The model under review builds one solid part; all positions refer to its coordinate system, in mm. A direction names the side the tool comes from. Round coordinates to 2 decimals unless told otherwise and drop trailing zeros. Order: outer loops, then holes, each group sorted by start corner. A loop starts at its lowest first (then second) coordinate and runs counter-clockwise, first axis right, second up. Notation, with made-up numbers: M -36.5,-34 L -2.5,-34 A27 cw -2.5,-18 Z; hole C -35,36.25 d6. An arc over 180 degrees is marked long. Answer as a JSON object with one key per item and string values. Group by question number.
1) The part is to be moulded in two halves that separate along X. For faces 3 (the cylindrical face through (12.932, -5.362, 76.415)), 4 (the cylindrical face through (-6.1, -0.2, 22.64)), 5 (the flat face through (0, 0, 0)), say which applies: +X half, -X half, draft (parallel to the pull), parting line (faces both ways), or undercut.
2) For faces 1 (the cylindrical face through (-2.17, -9.76, 167.32)), 2 (the flat face through (0, 0, 210)), list the 3-axis set-ups (+Z, -Z, +X, -X, +Y, -Y) from which the entire face can be reached by the end or side of a thin tool; tool diameter is ignored.
3) Consider section C-C, the plane z = 147. Write out the cut boundary in (x, y), then the cut area to 3 significant figures.
4) Consider section A-A, the plane x = 0. Write out the cut boundary in (y, z), then the cut area to 3 significant figures.
5) To check wall thickness, follow line 1 (Z direction, x = -1.5, y = -1.5); line 2 (Z direction, x = -1.75, y = -12.5); line 3 (X direction, y = 11.25, z = 19.5). State the ranges of each line that lie inside material, in increasing order.
6) Consider section B-B, the plane y = 5. Write out the cut boundary in (x, z) (3 decimals), then the cut area to 3 significant figures.
7) Consider section D-D, the plane y = -4.5. Write out the cut boundary in (x, z), then the cut area to 3 significant figures.
8) Insertion check: pin 1 Ø6 at (x, z) = (-6, 39.5) entering from +Y; pin 2 Ø6 at (x, z) = (8.5, 99) entering from +Y; pin 3 Ø1.5 at (x, z) = (6.5, 184) entering from -Y; pin 4 Ø10.5 at (x, z) = (0.39, 22.24) entering from -Y. Each pin has a flat end and moves straight along its axis. Give the tip position at first contact, or say it passes through.
```python
from build123d import *

# Parameters (mm, degrees)
SKETCH_R     = 14
PAD_DEPTH    = 155
SKETCH001_R  = 10
PAD001_DEPTH = 25
SKETCH002_R  = 8
PAD002_DEPTH = 30
SKETCH003_R  = 6.5
POCKET_DEPTH = 14


with BuildPart() as part:
    # Sketch → Pad (new body)
    with BuildSketch(Plane.XY):
        Circle(SKETCH_R)
    extrude(amount=PAD_DEPTH)

    # Sketch001 (on Face3 of Pad) → Pad001 (join)
    with BuildSketch(Plane.XY.offset(155)):
        Circle(SKETCH001_R)
    extrude(amount=PAD001_DEPTH)

    # Sketch002 (on Face5 of Pad001) → Pad002 (join)
    with BuildSketch(Plane.XY.offset(180)):
        Circle(SKETCH002_R)
    extrude(amount=PAD002_DEPTH)

    # Sketch003 (on DatumPlane) → Pocket (cut, symmetric)
    with BuildSketch(Plane(origin=(0, 0, 210), x_dir=(0.999848, 0, -0.017452), z_dir=(0, -1, 0))):
        with Locations((3.662873, -187.723682)):
            Circle(SKETCH003_R)
    extrude(amount=POCKET_DEPTH, both=True, mode=Mode.SUBTRACT)


solid = part.part
```
Results list:
{
 "1": {"face 3": "parting line", "face 4": "undercut", "face 5": "draft"},
 "2": {"face 1": "+Z", "face 2": "+Z, +X, -X, +Y, -Y"},
 "3": {"outline": "C 0,0 d28", "area": "616 mm^2"},
 "4": {"outline": "M -14,0 L 14,0 L 14,15.75 L -14,15.75 Z; M -14,28.73 L 14,28.73 L 14,155 L 10,155 L 10,180 L 8,180 L 8,210 L -8,210 L -8,180 L -10,180 L -10,155 L -14,155 Z", "area": "4,960 mm^2"},
 "5": {"line 1": "0 to 16.02, 28.46 to 210", "line 2": "0 to 16.1, 28.38 to 155", "line 3": "-8.33 to -5.51, 6.28 to 8.33"},
 "6": {"outline": "M -13.077,0 L 13.077,0 L 13.077,155 L 8.66,155 L 8.66,180 L 6.245,180 L 6.245,210 L -6.245,210 L -6.245,180 L -8.66,180 L -8.66,155 L -13.077,155 Z; hole C 0.386,22.241 d13", "area": "4,730 mm^2"},
 "7": {"outline": "M -13.26,0 L 13.26,0 L 13.26,155 L 8.93,155 L 8.93,180 L 6.61,180 L 6.61,210 L -6.61,210 L -6.61,180 L -8.93,180 L -8.93,155 L -13.26,155 Z; hole C 0.39,22.24 d13", "area": "4,820 mm^2"},
 "8": {"pin 1": "y = 13.67", "pin 2": "y = 12.87", "pin 3": "y = -5.56", "pin 4": "through"}
}
